Geometry check sheet. Reference: the model listing, model coordinates, mm. A direction names the side the tool comes from. Give positions to 0.01 mm unless a question says otherwise; leave off trailing zeros. Loops run counter-clockwise (first coordinate to the right, second up) from the corner with the lowest first, then second, coordinate; pieces in that order, holes last. Notation, with made-up numbers: (-4.5, 58.25) - (36.5, 58.25) arc R21 ccw to (36.5, 71.25) - close; hole circle Ø4 at (63, 63). An arc over 180 degrees is marked (long way). Use a Markdown table: item, result. Add a question column.
1. Material ranges on L1, parallel to Y at x = -4.75, z = 5.5 (3 decimals); L2, parallel to X at y = -39.5, z = 0 (3 decimals); L3, parallel to X at y = -8, z = 0 (3 decimals), recorded low to high.
2. Set-up check for faces 1 (the cylindrical face through (-3.49, -52.29, 3.86)), 2 (the cylindrical face through (-2.08, -10.31, 6.6)), 3 (the cylindrical face through (-0.306, -13.012, -6.102)), 4 (the flat face through (-4, -57, -2.794)), 5 (the flat face through (7, -7.493, 2)): record each of +Z, -Z, +X, -X, +Y, -Y from which the full face is reachable in a straight line by a thin tool's end or side.
3. Draft check along Z on faces 6 (the flat face through (4, -57, -2.794)), 7 (the cylindrical face through (-2.08, -1.16, 6.6)), 8 (the flat face through (4, -4.572, 5)). Enter one of: pulls with the +Z half, pulls with the -Z half, needs draft (parallel to the pull), parting line crosses it, or undercut.
4. Cross-section at C-C on y = -20.5. Enter the section's corners in (x, z), and give its area (3 significant figures).
5. Cross-section at B-B on y = -36.5. Enter the section's corners in (x, z) (3 decimals), and give its area (3 significant figures).
6. Cross-section at A-A on y = -49.53. Enter the section's corners in (x, z) (3 decimals), and give its area (3 significant figures).
7. Depth check by flat-ended pin: P1, Ø5.5, axis at x = 0, z = 0, coming from the -Y side; P2, Ø1.2, axis at x = -4.5, y = -57.5, coming from the +Z side; P3, Ø1.5, axis at x = 0.5, y = -32.5, coming from the -Z side; P4, Ø0.6, axis at x = 5.5, y = -56.5, coming from the -Z side. Enter the tip coordinate at first touch or a pass-through.
from build123d import *

# Parameters (mm, degrees)
SKETCH3_W                        = 1.0795
SKETCH3_H                        = 2.286
SKETCH4_W                        = 1.3335
SKETCH4_H                        = 1.016
SKETCH6_R                        = 3.937
AIR_OUT_2_MOUTHPIECE_DEPTH       = 60.575048888
SKETCH7_R                        = 2.3495
AIR_OUT_2_BC_DEPTH               = 60.575048986
SKETCH8_R                        = 1.27
VENT_DEPTH                       = 60.575048986
SLOT_FOR_DEMAND_LEVER_DEPTH      = 60.575048986
SLOT_FOR_DEMAND_LEVER_DEPTH_BACK = 60.575048986
SKETCH9_W                        = 3.048
SKETCH9_H                        = 2.54
SKETCH10_W                       = 16.383
SKETCH10_H                       = 2.4765
CLOCKING_CUT_DEPTH               = 2.54
SKETCH11_R                       = 4.445
SKETCH11_R_2                     = 3.175
SPRING_REST_DEPTH                = 1.27


with BuildPart() as part:
    # Sketch2 → Main Shaft (revolve)
    with BuildSketch(Plane.XY, mode=Mode.PRIVATE) as main_shaft_sk:
        Polygon((0, 0), (6.9215, 0), (6.9215, -12.065), (8.1915, -12.065), (8.1915, -18.923), (6.9215, -18.923), (6.9215, -22.86), (8.1915, -22.86), (8.1915, -35.56), (5.715, -35.56), (5.715, -58.42), (0, -58.42), align=None)
    revolve(main_shaft_sk.sketch.rotate(Axis((0, 0, 0), (0, -1, 0)), 90), axis=Axis((0, 0, 0), (0, -1, 0)))

    # Sketch3 → Top Groove (revolve, cut)
    with BuildSketch(Plane.XY, mode=Mode.PRIVATE) as top_groove_sk:
        with Locations((6.38175, -3.429)):
            Rectangle(SKETCH3_W, SKETCH3_H)
    revolve(top_groove_sk.sketch.rotate(Axis((0, 0, 0), (0, -1, 0)), 90), axis=Axis((0, 0, 0), (0, -1, 0)), mode=Mode.SUBTRACT)

    # Sketch4 → Upper Flange (revolve)
    with BuildSketch(Plane.XY, mode=Mode.PRIVATE) as upper_flange_sk:
        with Locations((7.58825, -8.001)):
            Rectangle(SKETCH4_W, SKETCH4_H)
    revolve(upper_flange_sk.sketch.rotate(Axis((0, 0, 0), (0, -1, 0)), 90), axis=Axis((0, 0, 0), (0, -1, 0)))

    # Sketch5 → ID 2 (revolve, cut)
    with BuildSketch(Plane.XY, mode=Mode.PRIVATE) as id_2_sk:
        Polygon((0, 0), (4.699, 0), (4.699, -23.359316239), (4.445, -23.359316239), (4.445, -58.42), (0, -58.42), align=None)
    revolve(id_2_sk.sketch.rotate(Axis((0, 0, 0), (0, -1, 0)), 90), axis=Axis((0, 0, 0), (0, -1, 0)), mode=Mode.SUBTRACT)

    # Sketch6 → Air Out 2 Mouthpiece (cut, through all)
    with BuildSketch(Plane.XY):
        with Locations(Location((0, -50.4698, 0), (0, 0, 270))):
            Circle(SKETCH6_R)
    extrude(amount=AIR_OUT_2_MOUTHPIECE_DEPTH, mode=Mode.SUBTRACT)

    # Sketch7 → Air Out 2 BC (cut, through all)
    with BuildSketch(Plane.XY):
        with Locations((0, -15.3416)):
            Circle(SKETCH7_R)
    extrude(amount=-AIR_OUT_2_BC_DEPTH, mode=Mode.SUBTRACT)

    # Sketch8 → Vent (cut, through all)
    with BuildSketch(Plane.XY):
        with Locations((0, -49.53)):
            Circle(SKETCH8_R)
    extrude(amount=-VENT_DEPTH, mode=Mode.SUBTRACT)

    # Sketch9 → Slot for Demand Lever (cut, two sides: drawn at the far end of the back side and taken through both)
    with BuildSketch(Plane(origin=(0, 0, 0), x_dir=(0, 0, -1), z_dir=(1, 0, 0)).offset(-SLOT_FOR_DEMAND_LEVER_DEPTH_BACK)):
        with Locations((1.27, -57.15)):
            Rectangle(SKETCH9_W, SKETCH9_H)
    extrude(amount=SLOT_FOR_DEMAND_LEVER_DEPTH + SLOT_FOR_DEMAND_LEVER_DEPTH_BACK, mode=Mode.SUBTRACT)

    # Sketch10 → Clocking cut (cut)
    with BuildSketch(Plane.XZ.offset(35.56)):
        with Locations((0, -6.95325)):
            Rectangle(SKETCH10_W, SKETCH10_H)
    extrude(amount=-CLOCKING_CUT_DEPTH, mode=Mode.SUBTRACT)

    # Sketch11 → Spring Rest (add)
    with BuildSketch(Plane.XZ.offset(55.88)):
        with Locations(Location((0, 0, 0), (0, 0, 90))):
            Circle(SKETCH11_R)
        with Locations(Location((0, 0, 0), (0, 0, 270))):
            Circle(SKETCH11_R_2, mode=Mode.SUBTRACT)
    extrude(amount=-SPRING_REST_DEPTH)


solid = part.part
Values found:
| question | item | result |
|---|---|---|
| 1 | L1 | y = -35.56 to -22.86, -18.923 to -12.065, -8.509 to -7.493 |
| 1 | L2 | x = -5.715 to -4.445, 4.445 to 5.715 |
| 1 | L3 | x = -8.255 to -4.699, 4.699 to 8.255 |
| 2 | face 1 | +Z |
| 2 | face 2 | none |
| 2 | face 3 | -Z |
| 2 | face 4 | +X, -X, -Y |
| 2 | face 5 | +Y |
| 3 | face 6 | undercut |
| 3 | face 7 | parting line crosses it |
| 3 | face 8 | needs draft |
| 4 | outline | circle Ø13.84 at (0, 0); hole circle Ø9.4 at (0, 0) |
| 4 | area | 81.1 mm2 |
| 5 | outline | circle Ø11.43 at (0, 0); hole circle Ø8.89 at (0, 0) |
| 5 | area | 40.5 mm2 |
| 6 | outline | (-3.823, 2.267) - (-3.823, 4.248) arc R5.715 ccw to (-1.27, -5.572) - (-1.27, -4.26) arc R4.445 cw to start; (1.27, -5.572) arc R5.715 ccw to (3.823, 4.248) - (3.823, 2.267) arc R4.445 cw to (1.27, -4.26) - close |
| 6 | area | 26.2 mm2 |
| 7 | P1 | passes through |
| 7 | P2 | stops at z = 4.18 |
| 7 | P3 | stops at z = -8.19 |
| 7 | P4 | stops at z = 0.25 |
